```python
from build123d import *

# Parameters (mm, degrees)
SKETCH1_R           = 37.5
SKETCH1_R_2         = 7.2
SKETCH1_R_3         = 1.5
BOSS_EXTRUDE1_DEPTH = 4
SKETCH2_R           = 11.2
SKETCH2_R_2         = 7.2
BOSS_EXTRUDE2_DEPTH = 8


with BuildPart() as part:
    # Sketch1 → Boss-Extrude1 (new body)
    with BuildSketch(Plane.XY):
        Circle(SKETCH1_R)
        Circle(SKETCH1_R_2, mode=Mode.SUBTRACT)
        with Locations((22.5, 0)):
            Circle(SKETCH1_R_3, mode=Mode.SUBTRACT)
        with Locations((-11.25, -19.485571585)):
            Circle(SKETCH1_R_3, mode=Mode.SUBTRACT)
        with Locations((-11.25, 19.485571585)):
            Circle(SKETCH1_R_3, mode=Mode.SUBTRACT)
        with Locations((21.213203436, 21.213203436)):
            Circle(SKETCH1_R_3, mode=Mode.SUBTRACT)
        with Locations((21.213203436, -21.213203436)):
            Circle(SKETCH1_R_3, mode=Mode.SUBTRACT)
        with Locations((-21.213203436, -21.213203436)):
            Circle(SKETCH1_R_3, mode=Mode.SUBTRACT)
        with Locations((-21.213203436, 21.213203436)):
            Circle(SKETCH1_R_3, mode=Mode.SUBTRACT)
    extrude(amount=BOSS_EXTRUDE1_DEPTH)

    # Sketch2 → Boss-Extrude2 (add)
    with BuildSketch(Plane(origin=(0, 0, 0), x_dir=(-1, 0, 0), z_dir=(0, 0, -1))):
        Circle(SKETCH2_R)
        Circle(SKETCH2_R_2, mode=Mode.SUBTRACT)
    extrude(amount=BOSS_EXTRUDE2_DEPTH)


solid = part.part
```
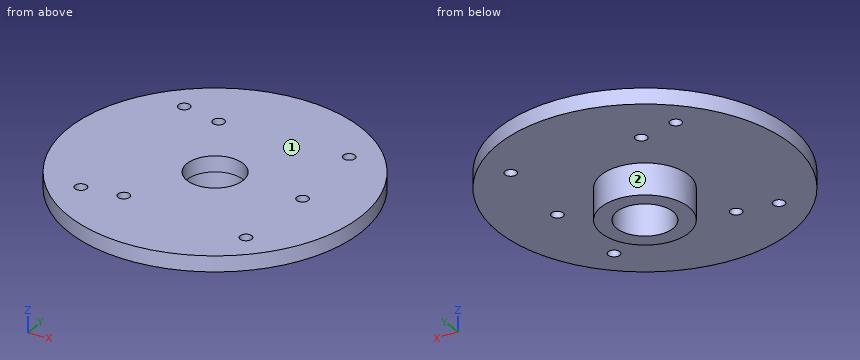
Part model, mm, in its own coordinate system. Face numbers are marked on the shaded views. A direction names the side the tool comes from. Round coordinates to 2 decimals unless told otherwise and drop trailing zeros. Order: outer loops, then holes, each group sorted by start corner. A loop starts at its lowest first (then second) coordinate and runs counter-clockwise, first axis right, second up. Notation, with made-up numbers: M 12,29 L 66,29 A5 cw 66,37 Z; hole C 88,23.5 d1. An arc over 180 degrees is marked long. Put each result on its own line as item: value. Start each with the question number.
1. Slice it at A-A on y = 0. List the corners of the cut face in (x, z).
2. Slice it at D-D on x = 28. List the corners of the cut face in (y, z).
3. Drill centre lines: probe 1 along Y at (x, z) = (20, 1); probe 2 along Y at (x, z) = (22, 1); probe 3 along Y at (x, z) = (22.5, 2.1). Where is each one in solid material? Low to high. Write a range as [from, to].
4. Slice it at B-B on x = 0. List the corners of the cut face in (y, z), then the cut area to 3 significant figures.
5. Tool access for the marked faces 1 and 2: list every direction of +Z, -Z, +X, -X, +Y, -Y with a clear straight run to the whole face (end or side of a thin tool).
6. Drop flat-ended pins along their axis: pin 1 (6 mm diameter, centred on x = 24, z = 0, fed in from +Y); pin 2 (11.5 mm diameter, centred on x = 0, y = 0, fed in from +Z); pin 3 (5 mm diameter, centred on y = -3, z = -2, fed in from +X); pin 4 (22.5 mm diameter, centred on x = 11.5, y = 17, fed in from -Z). Give the stop position or say it passes through.
7. Slice it at C-C on y = -9. List the corners of the cut face in (x, z).
Findings:
1. outline: M -37.5,0 L -11.2,0 L -11.2,-8 L -7.2,-8 L -7.2,4 L -37.5,4 Z; M 7.2,-8 L 11.2,-8 L 11.2,0 L 21,0 L 21,4 L 7.2,4 Z; M 24,0 L 37.5,0 L 37.5,4 L 24,4 Z
2. outline: M -24.94,0 L 24.94,0 L 24.94,4 L -24.94,4 Z
3. probe 1: [-31.72, -22.1], [-20.33, 20.33], [22.1, 31.72]
3. probe 2: [-30.37, -22.49], [-19.94, -1.41], [1.41, 19.94], [22.49, 30.37]
3. probe 3: [-30, -21.98], [-20.44, -1.5], [1.5, 20.44], [21.98, 30]
4. outline: M -37.5,0 L -11.2,0 L -11.2,-8 L -7.2,-8 L -7.2,4 L -37.5,4 Z; M 7.2,-8 L 11.2,-8 L 11.2,0 L 37.5,0 L 37.5,4 L 7.2,4 Z
4. area: 306 mm2
5. face 1: +Z, +X, -X, +Y, -Y
5. face 2: -Z
6. pin 1: y = 31.07
6. pin 2: through
6. pin 3: x = 37.47
6. pin 4: z = -8
7. outline: M -36.4,0 L -6.67,0 L -6.67,-8 L 6.67,-8 L 6.67,0 L 36.4,0 L 36.4,4 L -36.4,4 Z
